from build123d import *

# Parameters (mm, degrees)
BOSS_EXTRUDE1_DEPTH  = 12.5
FILLET1_R            = 12.5
SKETCH2_R            = 2.5
CUT_EXTRUDE1_DEPTH   = 45.370598373
FILLET1_OF_MIRROR1_R = 12.5


with BuildPart() as part:
    # Sketch1 → Boss-Extrude1 (new, symmetric)
    with BuildSketch(Plane(origin=(0, 0, 0), x_dir=(1, 0, 0), z_dir=(0, 1, 0))):
        Polygon((26, -31), (26, 32.5), (27.5, 32.5), (27.5, -32.5), (-27.5, -32.5), (-27.5, 32.5), (-26, 32.5), (-26, -31), align=None)
    boss_extrude1 = extrude(amount=BOSS_EXTRUDE1_DEPTH, both=True)

    # Fillet1
    fillet1_edges = [part.edges().sort_by_distance(p)[0] for p in [
        (-26.75, -12.5, -32.5),
        (-26.75, 12.5, -32.5),
        (26.75, -12.5, -32.5),
        (26.75, 12.5, -32.5),
    ]]
    fillet(fillet1_edges, radius=FILLET1_R - 0.0001)  # a hair under: the kernel refuses the full size

    # Sketch2 → Cut-Extrude1 (cut, symmetric)
    with BuildSketch(Plane(origin=(0, 0, 0), x_dir=(0, 0, -1), z_dir=(1, 0, 0))):
        with Locations((20, 0)):
            Circle(SKETCH2_R)
    cut_extrude1 = extrude(amount=CUT_EXTRUDE1_DEPTH, both=True, mode=Mode.SUBTRACT)

    # Mirror1: Boss-Extrude1, Cut-Extrude1 across plane
    add(boss_extrude1.mirror(Plane(origin=(27.5, 12.5, 32.5), x_dir=(1, 0, 0), z_dir=(0, 0, -1))))
    add(cut_extrude1.mirror(Plane(origin=(27.5, 12.5, 32.5), x_dir=(1, 0, 0), z_dir=(0, 0, -1))), mode=Mode.SUBTRACT)

    # Fillet1 of Mirror1
    fillet1_of_mirror1_edges = [part.edges().sort_by_distance(p)[0] for p in [
        (-26.75, -12.5, 97.5),
        (-26.75, 12.5, 97.5),
        (26.75, -12.5, 97.5),
        (26.75, 12.5, 97.5),
    ]]
    fillet(fillet1_of_mirror1_edges, radius=FILLET1_OF_MIRROR1_R - 0.0001)  # a hair under: the kernel refuses the full size


solid = part.part
Read the model definition and answer for the solid it produces. Units are mm, in the model's axes. A direction names the side the tool comes from. Coordinates: 2 decimals unless noted, no trailing zeros. Loops run counter-clockwise (first coordinate to the right, second up) from the corner with the lowest first, then second, coordinate; pieces in that order, holes last. Notation, with made-up numbers: (37, 57.5) - (51, 57.5) arc R16 cw to (51, 88.5) - close; hole circle Ø3 at (66.25, -10.75). An arc over 180 degrees is marked (long way). Answer in a Markdown table with one row per item.
Q1. Find section B-B on y = 6.5. Write down the section's boundary in (x, z).
Here are the results:
| item | result |
|---|---|
| outline | (-27.5, -30.68) - (-26, -30.68) - (-26, 31) - (26, 31) - (26, -30.68) - (27.5, -30.68) - (27.5, 95.68) - (26, 95.68) - (26, 34) - (-26, 34) - (-26, 95.68) - (-27.5, 95.68) - close |
Q2. Given P1, Ø1.5, axis at x = 4, y = -3.5, coming from the -Z side; P2, Ø5, axis at x = -1.5, y = -8, coming from the +Z side, each flat-ended and moving along its own axis, determine where each tip first touches the part or whether it passes through.
Here are the results:
| item | result |
|---|---|
| P1 | stops at z = 31 |
| P2 | stops at z = 34 |
Q3. The mould has two halves that part along X. Classify faces 1 (the cylindrical face through (-26.7, 0.1, 82.5)), 2 (the flat face through (-26, 0, 66)), 3 (the flat face through (-27.5, 0, 32)): pulls with the +X half, pulls with the -X half, needs draft (parallel to the pull), parting line crosses it, or undercut.
Here are the results:
| item | result |
|---|---|
| face 1 | needs draft |
| face 2 | undercut |
| face 3 | pulls with the -X half |
Q4. For faces 4 (the flat face through (26, 0, 65)), 5 (the flat face through (0, 12.5, 33)), 6 (the flat face through (26, 0, 0)), determine the directions among +Z, -Z, +X, -X, +Y, -Y from which every point of the face is accessible in a straight line to the end or side of a thin tool.
Here are the results:
| item | result |
|---|---|
| face 4 | +Z, +Y, -Y |
| face 5 | +Z, -Z, +X, -X, +Y |
| face 6 | -Z, +Y, -Y |
Q5. Find section A-A on z = 81. Write down the section's boundary in (x, y), plus the area to 3 significant figures.
Here are the results:
| item | result |
|---|---|
| outline | (-27.5, -12.5) - (-26, -12.5) - (-26, 12.5) - (-27.5, 12.5) - close; (26, -12.5) - (27.5, -12.5) - (27.5, 12.5) - (26, 12.5) - close |
| area | 75.0 mm^2 |
Q6. Straight lines are drawn through the part: line 1 along X through (y, z) = (11, 36.5); line 2 along Y through (x, z) = (27, 85); line 3 along Z through (x, y) = (7, -5.75). For each, find the intervals that lie inside material, in ascending order. Write a range as [from, to].
Here are the results:
| item | result |
|---|---|
| line 1 | x = [-27.5, -26], [26, 27.5] |
| line 2 | y = [-12.5, -2.5], [2.5, 12.5] |
| line 3 | z = [31, 34] |
Q7. Find section C-C on x = 14. Write down the section's boundary in (y, z).
Here are the results:
| item | result |
|---|---|
| outline | (-12.5, 31) - (12.5, 31) - (12.5, 34) - (-12.5, 34) - close |
Q8. Find section D-D on y = -7. Write down the section's boundary in (x, z).
Here are the results:
| item | result |
|---|---|
| outline | (-27.5, -30.36) - (-26, -30.36) - (-26, 31) - (26, 31) - (26, -30.36) - (27.5, -30.36) - (27.5, 95.36) - (26, 95.36) - (26, 34) - (-26, 34) - (-26, 95.36) - (-27.5, 95.36) - close |
